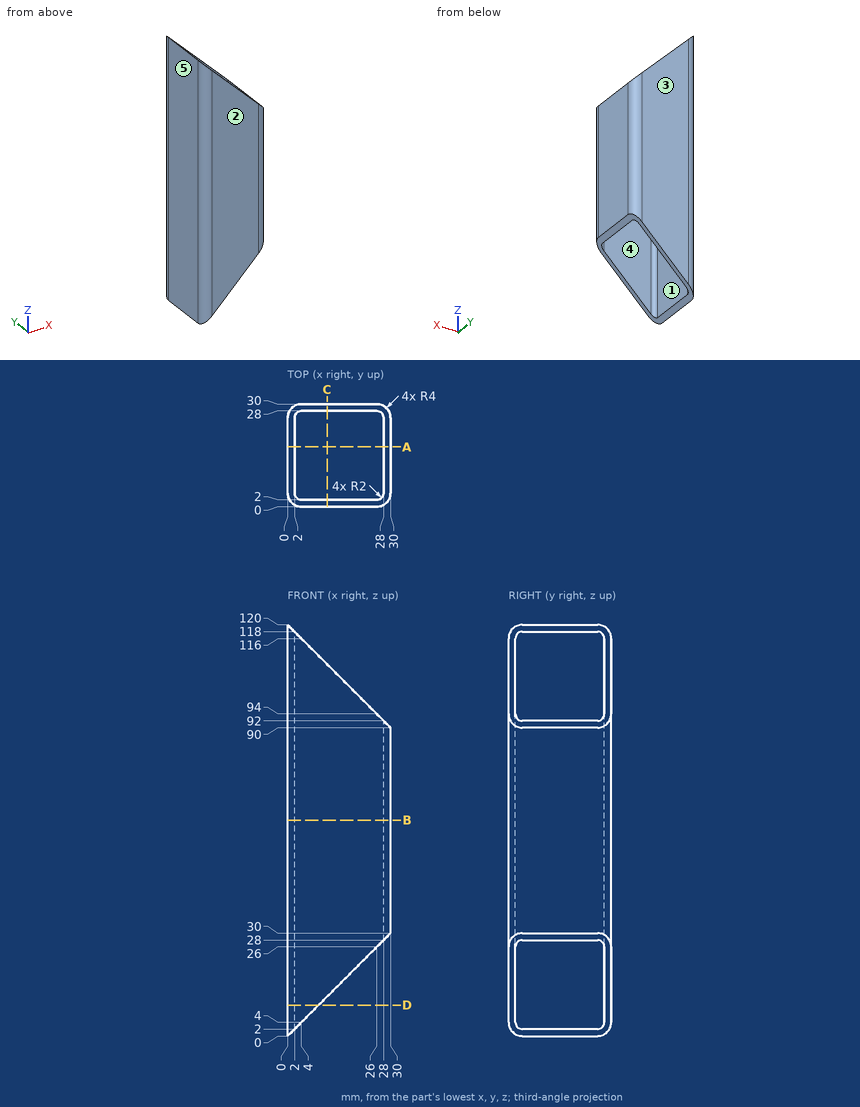
Part print with two shaded views. Sizes in mm from the minimum x, y, z corner. A direction names the side the tool comes from. Round coordinates to 2 decimals unless told otherwise and drop trailing zeros. Loops run counter-clockwise (first coordinate to the right, second up) from the corner with the lowest first, then second, coordinate; pieces in that order, holes last. Notation, with made-up numbers: (53, 16.5) - (61, 16.5) arc R21 ccw to (61, 38.5) - close; hole circle Ø5 at (-16.5, -35.75). An arc over 180 degrees is marked (long way). Put each result on its own line as item: value.
1. Slice it at A-A on y = 17.5. List the corners of the cut face in (x, z).
Geometry check:
outline: (0, 0) - (2, 2) - (2, 118) - (0, 120) - close; (28, 28) - (30, 30) - (30, 90) - (28, 92) - close
2. Slice it at B-B on z = 63. List the corners of the cut face in (x, y).
Geometry check:
outline: (0, 4) arc R4 ccw to (4, 0) - (26, 0) arc R4 ccw to (30, 4) - (30, 26) arc R4 ccw to (26, 30) - (4, 30) arc R4 ccw to (0, 26) - close; hole (2, 4) arc R2 ccw to (4, 2) - (26, 2) arc R2 ccw to (28, 4) - (28, 26) arc R2 ccw to (26, 28) - (4, 28) arc R2 ccw to (2, 26) - close
3. Wall check: line 1 (X direction, y = 24.75, z = 40); line 2 (Y direction, x = 26.5, z = 74.5). Give the ranges that are in metal, low to high.
Geometry check:
line 1: 0 to 2, 28 to 30
line 2: 0.03 to 2.06, 27.94 to 29.97
4. Two-plate mould, pull along Y, no slides. Class the marked faces 1, 2 and 3: released by +Y, released by -Y, zero draft, split by the parting line, or undercut.
Geometry check:
face 1: undercut
face 2: released by -Y
face 3: released by +Y
5. 3-axis set-ups, long thin cutter, end or side, ignore diameter. For the marked faces 4 and 5: which of +Z, -Z, +X, -X, +Y, -Y reach the whole face in a straight line?
Geometry check:
face 4: +Z, -Z
face 5: +Z, -Z, -X, +Y, -Y
6. Slice it at D-D on z = 9. List the corners of the cut face in (x, y).
Geometry check:
outline: (0, 4) arc R4 ccw to (4, 0) - (9, 0) - (9, 2) - (4, 2) arc R2 cw to (2, 4) - (2, 26) arc R2 cw to (4, 28) - (9, 28) - (9, 30) - (4, 30) arc R4 ccw to (0, 26) - close
7. Slice it at C-C on x = 11.5. List the corners of the cut face in (y, z), and give its area (3 significant figures).
Geometry check:
outline: (0, 11.5) - (2, 11.5) - (2, 108.5) - (0, 108.5) - close; (28, 11.5) - (30, 11.5) - (30, 108.5) - (28, 108.5) - close
area: 388 mm²
